```python
from build123d import *

# Parameters (mm, degrees)
F0_R     = 15.875
F1_DEPTH = 1.778
F3_R     = 0.889
F4_DEPTH = 1.91313
F5_R     = 1.524
F5_W     = 3.048
F5_H     = 6.400035
F6_DEPTH = 2.22015


with BuildPart() as f1:
    # F0 (on Top) → F1 (new body)
    with BuildSketch(Plane.XY):
        Circle(F0_R)
    extrude(amount=-F1_DEPTH)

    # F3 (on face) → F4 (cut)
    with BuildSketch(Plane.XY):
        with Locations((0, 13.652203)):
            Circle(F3_R)
        with Locations((-13.659894, -0.015021)):
            Circle(F3_R)
        with Locations((13.674476, -0.124876)):
            Circle(F3_R)
    extrude(amount=-F4_DEPTH, mode=Mode.SUBTRACT)

    # F5 (on face) → F6 (cut)
    with BuildSketch(Plane.XY):
        Circle(F5_R)
        with Locations((0, 5.805492)):
            Rectangle(F5_W, F5_H)
    extrude(amount=-F6_DEPTH, mode=Mode.SUBTRACT)


solid = f1.part
```
Build history of the part. All positions in model axes, mm. A direction names the side the tool comes from. Round coordinates to 2 decimals unless told otherwise and drop trailing zeros. Order: outer loops, then holes, each group sorted by start corner. A loop starts at its lowest first (then second) coordinate and runs counter-clockwise, first axis right, second up. Notation, with made-up numbers: (53, 26.5) -> (93, 26.5) arc R15 ccw to (93, 54.5) -> close; hole circle Ø9 at (81.25, 24). An arc over 180 degrees is marked (long way). Answer in a Markdown table with one row per item.
1) Band-saw the part on B-B on z = -0.6. Give the number of separate pieces and of enclosed holes in the cut face, and give its area (3 significant figures).
Values:
| item | result |
|---|---|
| separate pieces | 1 |
| enclosed holes | 5 |
| area | 757 mm2 |
2) Mould opens along Y. For faces 1 (the cylindrical face through (-3.441, -15.497, -0.877)), 2 (the cylindrical face through (-12.81, 0.25, -0.88)), 3 (the flat face through (0, -3, 0)) say: released by +Y, released by -Y, zero draft, split by the parting line, or undercut.
Values:
| item | result |
|---|---|
| face 1 | split by the parting line |
| face 2 | undercut |
| face 3 | zero draft |
3) Band-saw the part on C-C on x = -10.5. Give the cut face in (y, z), and give its area (3 significant figures).
Values:
| item | result |
|---|---|
| outline | (-11.91, -1.78) -> (11.91, -1.78) -> (11.91, 0) -> (-11.91, 0) -> close |
| area | 42.3 mm2 |
4) Band-saw the part on D-D on y = -9. Give the cut face in (x, z), and give its area (3 significant figures).
Values:
| item | result |
|---|---|
| outline | (-13.08, -1.78) -> (13.08, -1.78) -> (13.08, 0) -> (-13.08, 0) -> close |
| area | 46.5 mm2 |
5) Wall check: L1, parallel to Y at x = 0, z = -1 (1 decimal); L2, parallel to X at y = 0.5, z = -1.7; L3, parallel to X at y = 7.5, z = -0.6. Give the ranges that are in metal, low to high.
Values:
| item | result |
|---|---|
| L1 | -15.9 to -1.5, 1.5 to 2.6, 9 to 12.8, 14.5 to 15.9 |
| L2 | -15.87 to -14.38, -12.94 to -1.44, 1.44 to 13.04, 14.31 to 15.87 |
| L3 | -13.99 to -1.52, 1.52 to 13.99 |
6) Band-saw the part on A-A on x = 0. Give the cut face in (y, z) (1 decimal), and give its area (3 significant figures).
Values:
| item | result |
|---|---|
| outline | (-15.9, -1.8) -> (-1.5, -1.8) -> (-1.5, 0) -> (-15.9, 0) -> close; (1.5, -1.8) -> (2.6, -1.8) -> (2.6, 0) -> (1.5, 0) -> close; (9, -1.8) -> (12.8, -1.8) -> (12.8, 0) -> (9, 0) -> close; (14.5, -1.8) -> (15.9, -1.8) -> (15.9, 0) -> (14.5, 0) -> close |
| area | 36.5 mm2 |
7) Which spindle directions (+Z, -Z, +X, -X, +Y, -Y) get a long thin tool onto all of the face, cutting with end or side? Do faces 4 (the flat face through (0, -3, -1.778)), 5 (the flat face through (-1.524, 6, -1)). Say none if no direction does.
Values:
| item | result |
|---|---|
| face 4 | -Z, +X, -X, +Y, -Y |
| face 5 | +Z, -Z |
